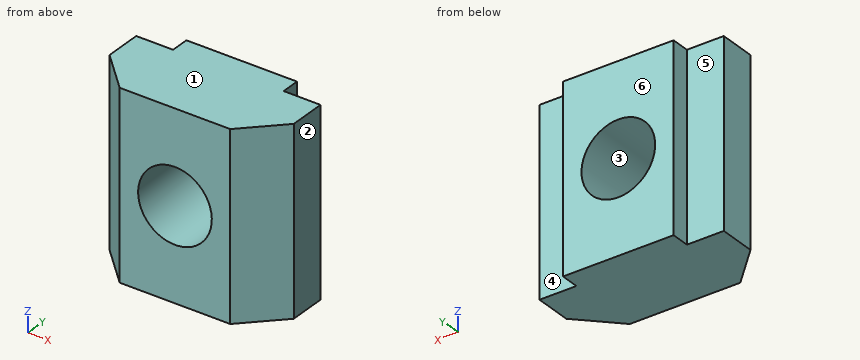
```python
from build123d import *

# Parameters (mm, degrees)
RESSALTO_EXTRUS_O1_DEPTH = 10
CHANFRO1_SIZE            = 2
ESBO_O2_R                = 2
CORTE_EXTRUS_O1_DEPTH    = 5


with BuildPart() as part:
    # Esboço1 → Ressalto-extrusão1 (new body)
    with BuildSketch(Plane.XY):
        Polygon((-3, 0), (3, 0), (3, -1), (5, -1), (5, -5), (-5, -5), (-5, -1), (-3, -1), align=None)
    extrude(amount=RESSALTO_EXTRUS_O1_DEPTH)

    # Chanfro1
    chanfro1_edges = [part.edges().sort_by_distance(p)[0] for p in [
        (5, -5, 5),
        (-5, -5, 5),
    ]]
    chamfer(chanfro1_edges, length=CHANFRO1_SIZE)

    # Esboço2 → Corte-extrusão1 (cut)
    with BuildSketch(Plane(origin=(0, 0, 0), x_dir=(1, 0, 0), z_dir=(0, 1, 0))):
        with Locations(Location((0, -5, 0), (0, 0, 270))):
            Circle(ESBO_O2_R)
    extrude(amount=-CORTE_EXTRUS_O1_DEPTH, mode=Mode.SUBTRACT)


solid = part.part
```
CAD build for the part. Positions are in the model's coordinates, mm. Face numbers are marked on the shaded views. A direction names the side the tool comes from. Coordinates: 2 decimals unless noted, no trailing zeros. Order: outer loops, then holes, each group sorted by start corner. A loop starts at its lowest first (then second) coordinate and runs counter-clockwise, first axis right, second up. Notation, with made-up numbers: M 89,64 L 119,64 A22 ccw 119,78 Z; hole C 26,42 d1. An arc over 180 degrees is marked long. Write each question's results on one line, items separated by ' | '. Start each with the question number.
Q1. Flat gauge pins, fed straight in: P1, Ø0.5, axis at y = -0.5, z = 7, coming from the +X side; P2, Ø2, axis at x = 4.5, z = 3.5, coming from the +Y side. Where does each tip first touch, or does it go through?
Q2. Cut at C-C (y = -2.35). List the corners of the cut face in (x, z), then the cut area to 3 significant figures.
Q3. Which spindle directions (+Z, -Z, +X, -X, +Y, -Y) get a long thin tool onto all of the face, cutting with end or side? Do the marked faces 4, 5 and 6. Say none if no direction does.
Q4. Cut at D-D (z = 2). List the corners of the cut face in (x, y).
Q5. Drill centre lines: probe 1 along X at (y, z) = (-2.95, 5); probe 2 along X at (y, z) = (-0.15, 4); probe 3 along Z at (x, y) = (0.25, -4.75). Where is each one in solid material? Low to high. Write a range as from..to.
Q6. Pull direction X, two halves, no side cores. Call the marked faces 1, 2 and 3: +X half, -X half, draft (parallel to the pull), parting line (faces both ways), or undercut.
Q7. Cut at A-A (x = 0). List the corners of the cut face in (y, z).
Q8. Cut at B-B (z = 5). List the corners of the cut face in (x, y).
Found:
1) P1: x = 3 | P2: y = -1
2) outline: M -5,0 L 5,0 L 5,10 L -5,10 Z; hole C 0,5 d4 | area: 87.4 mm²
3) face 4: +Z, -Z, +X, +Y | face 5: +Z, -Z, -X, +Y | face 6: +Z, -Z, +X, -X, +Y
4) outline: M -5,-3 L -3,-5 L 3,-5 L 5,-3 L 5,-1 L 3,-1 L 3,0 L -3,0 L -3,-1 L -5,-1 Z
5) probe 1: -5..-2, 2..5 | probe 2: -3..-1.73, 1.73..3 | probe 3: 0..3.02, 6.98..10
6) face 1: draft | face 2: +X half | face 3: undercut
7) outline: M -5,0 L 0,0 L 0,3 L -5,3 Z; M -5,7 L 0,7 L 0,10 L -5,10 Z
8) outline: M -5,-3 L -3,-5 L -2,-5 L -2,0 L -3,0 L -3,-1 L -5,-1 Z; M 2,-5 L 3,-5 L 5,-3 L 5,-1 L 3,-1 L 3,0 L 2,0 Z
